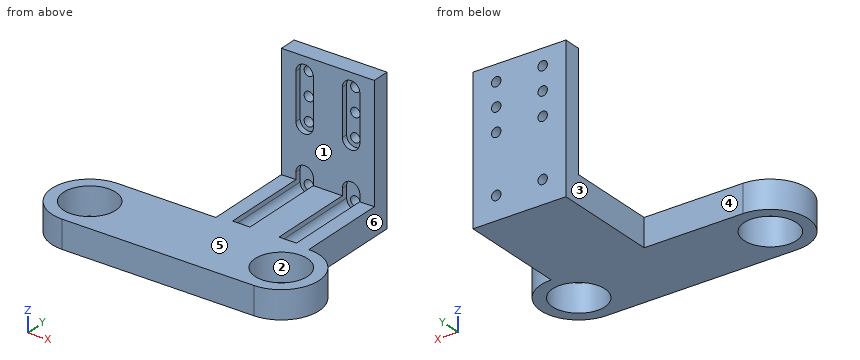
Autodesk Inventor part; units mm, degrees
ref_plane "Work Plane1" through (1.5875, 73.0746, 0) normal (0, 1, 0) x (1, 0, 0)
ref_plane "YZ Plane" through (0, 0, 0) normal (1, 0, 0) x (0, 1, 0)
ref_plane "XZ Plane" through (0, 0, 0) normal (0, 1, 0) x (-1, 0, 0)
sketch "Sketch1" plane through (0, 0, 0) normal (0, 0, 1) x (1, 0, 0)
  line L0 (-52.3875, 0) -> (52.3875, 0) construction
  line L1 (-52.3875, -20.6502) -> (52.3875, -20.6502)
  line L2 (52.3875, 20.6502) -> (-52.3875, 20.6502)
  arc A0 (-52.3875, 20.6502) -> (-52.3875, -20.6502) centre (-52.3875, 0) ccw
  arc A1 (52.3875, -20.6502) -> (52.3875, 20.6502) centre (52.3875, 0) ccw
  point P0 (0, 0)
  dimension "d0" = 104.775
  dimension "d1" = 20.6502
extrude "Extrusion1" add sketch "Sketch1" along normal blind 15.24
sketch "Sketch2" plane through (0, 0, 15.24) normal (0, 0, 1) x (1, 0, 0)
  arc A0 (-52.3875, 20.6502) -> (-52.3875, -20.6502) centre (-52.3875, 0) ccw
  circle A1 centre (-52.3875, 0) radius 14.3002
  arc A2 (52.3875, -20.6502) -> (52.3875, 20.6502) centre (52.3875, 0) ccw
  circle A3 centre (52.3875, 0) radius 14.3002
  point P0 (0, 0)
  dimension "d4" = 28.6004
extrude "Extrusion2" cut sketch "Sketch2" against normal through all
sketch "Sketch3" plane through (0, 0, 15.24) normal (0, 0, 1) x (1, 0, 0)
  line L0 (1.5875, 79.4246) -> (52.3875, 79.4246)
  line L1 (52.3875, 79.4246) -> (52.3875, 20.6502)
  line L2 (52.3875, 20.6502) -> (1.5875, 20.6502)
  line L3 (1.5875, 20.6502) -> (1.5875, 79.4246)
  line L4 (52.3875, 20.6502) -> (-52.3875, 20.6502)
  circle A0 centre (26.9875, 101.6496) radius 7.0281
  circle A1 centre (52.3875, 0) radius 14.3002
  point P0 (0, 0)
  point P1 (26.9875, 20.6502)
  point P2 (26.9875, 79.4246)
  dimension "d7" = 50.8
  dimension "d8" = 22.225
  dimension "d9" = 104.775
  dimension "d10" = 79.4246
extrude "Extrusion3" add sketch "Sketch3" against normal up to surface (15.24 mm away) contours L0 L1 L2 L3
sketch "Sketch4" plane through (0, 0, 15.24) normal (0, 0, 1) x (1, 0, 0)
  line L0 (1.5875, 79.4246) -> (1.5875, 20.6502)
  line L1 (1.5875, 79.4246) -> (52.3875, 79.4246)
  line L2 (52.3875, 79.4246) -> (52.3875, 69.8996)
  line L3 (52.3875, 69.8996) -> (1.5875, 69.8996)
  line L4 (1.5875, 69.8996) -> (1.5875, 79.4246)
  line L5 (52.3875, 20.6502) -> (52.3875, 79.4246)
  point P0 (0, 0)
  point P1 (25.4, 20.6502)
  dimension "d13" = 9.525
extrude "Extrusion4" add sketch "Sketch4" along normal blind 63.5
sketch "Sketch5" plane through (1.5875, 79.4246, 0) normal (0, 1, 0) x (1, 0, 0)
  circle A0 centre (38.1, -12.7) radius 2.5797
  line L0 (0, 0) -> (50.8, 0)
  line L1 (50.8, 0) -> (50.8, -78.74)
  circle A1 centre (12.7, -12.7) radius 2.5797
  circle A2 centre (38.1, -44.45) radius 2.5797
  circle A3 centre (12.7, -44.45) radius 2.5797
  circle A4 centre (38.1, -57.15) radius 2.5797
  circle A5 centre (12.7, -57.15) radius 2.5797
  circle A6 centre (38.1, -69.85) radius 2.5797
  circle A7 centre (12.7, -69.85) radius 2.5797
  line L2 (25.4, 0) -> (25.4, -6.0461)
  dimension "d17" = 5.1594
  dimension "d18" = 12.7
  dimension "d21" = 25.4
  dimension "d24" = 31.75
  dimension "d29" = 12.7
  dimension "d51" = 12.7
extrude "Extrusion5" cut sketch "Sketch5" against normal blind 50.8
ref_plane "Work Plane1" through (1.5875, 73.0746, 0) normal (0, 1, 0) x (1, 0, 0)
sketch "Sketch6" plane through (1.5875, 73.0746, 0) normal (0, 1, 0) x (1, 0, 0)
  line L0 (-53.975, 0) -> (50.8, 0)
  line L1 (50.8, -15.24) -> (50.8, -78.74)
  line L2 (38.1, -12.7) -> (38.1, -19.05) construction
  line L3 (33.3375, -12.7) -> (33.3375, -19.05)
  line L4 (42.8625, -19.05) -> (42.8625, -12.7)
  arc A0 (42.8625, -12.7) -> (33.3375, -12.7) centre (38.1, -12.7) ccw
  arc A1 (33.3375, -19.05) -> (42.8625, -19.05) centre (38.1, -19.05) ccw
  line L5 (12.7, -12.7) -> (12.7, -19.05) construction
  line L6 (7.9375, -12.7) -> (7.9375, -19.05)
  line L7 (17.4625, -19.05) -> (17.4625, -12.7)
  arc A2 (17.4625, -12.7) -> (7.9375, -12.7) centre (12.7, -12.7) ccw
  arc A3 (7.9375, -19.05) -> (17.4625, -19.05) centre (12.7, -19.05) ccw
  circle A4 centre (38.1, -44.45) radius 2.5797 construction
  circle A5 centre (38.1, -69.85) radius 2.5797 construction
  line L8 (38.1, -44.45) -> (38.1, -69.85) construction
  line L9 (33.3375, -44.45) -> (33.3375, -69.85)
  line L10 (42.8625, -69.85) -> (42.8625, -44.45)
  arc A6 (42.8625, -44.45) -> (33.3375, -44.45) centre (38.1, -44.45) ccw
  arc A7 (33.3375, -69.85) -> (42.8625, -69.85) centre (38.1, -69.85) ccw
  circle A8 centre (12.7, -44.45) radius 2.5797 construction
  circle A9 centre (12.7, -69.85) radius 2.5797 construction
  line L11 (12.7, -44.45) -> (12.7, -69.85) construction
  line L12 (7.9375, -44.45) -> (7.9375, -69.85)
  line L13 (17.4625, -69.85) -> (17.4625, -44.45)
  arc A10 (17.4625, -44.45) -> (7.9375, -44.45) centre (12.7, -44.45) ccw
  arc A11 (7.9375, -69.85) -> (17.4625, -69.85) centre (12.7, -69.85) ccw
  circle A12 centre (38.1, -12.7) radius 2.5797 construction
  circle A13 centre (12.7, -12.7) radius 2.5797 construction
  point P0 (-1.5875, 0)
  point P1 (38.1, -15.875)
  point P2 (12.7, -15.875)
  point P3 (38.1, -57.15)
  point P4 (12.7, -57.15)
  dimension "d47" = 6.35
  dimension "d48" = 4.7625
extrude "Extrusion6" cut sketch "Sketch6" against normal blind 50.8
properties part number "IntakeChainLinkVP"
Read the model definition and answer for the solid it produces. Units are mm, in the model's axes. Face numbers are marked on the shaded views. A direction names the side the tool comes from. Coordinates: 2 decimals unless noted, no trailing zeros. Write each loop counter-clockwise with the first axis right and the second up, starting at its lowest first coordinate (ties: lowest second). Pieces come first, ordered by that corner, then holes. Notation, with made-up numbers: (65.25, 55.25) - (78.25, 55.25) arc R19 ccw to (78.25, 92.25) - close; hole circle Ø7 at (-33, 6.25). An arc over 180 degrees is marked (long way). Answer as a JSON object with one key per item and string values. Group by question number.
1. A cutting plane is placed at A-A (y = 0). Determine the outline of the cut face in (x, z), plus the area to 3 significant figures.
2. Consider L1, parallel to X at y = 78, z = 44; L2, parallel to X at y = 76.25, z = 69.85; L3, parallel to Y at x = 18.5, z = 39. Determine where each line is inside the solid, lowest interval first. Write a range as [from, to].
3. Each of these flat-tipped pins is pushed along its axis until it touches: P1, Ø6.5, axis at x = 39.69, z = 69.85, coming from the -Y side; P2, Ø3, axis at y = 31.5, z = 13.5, coming from the -X side; P3, Ø1, axis at x = 32.5, z = 60.5, coming from the -Y side; P4, Ø3, axis at x = 13.5, z = 56.5, coming from the -Y side. Where does it stop, or does it pass through?
4. A cutting plane is placed at D-D (x = -15.5). Determine the outline of the cut face in (y, z), plus the area to 3 significant figures.
5. The mould has two halves that part along X. Classify the marked faces 1, 2 and 3: +X half, -X half, draft (parallel to the pull), parting line (faces both ways), or undercut.
6. A cutting plane is placed at B-B (z = 57.15). Give the number of separate pieces and of enclosed holes in the cut face, plus the area to 3 significant figures.
7. Which of the six approach directions +Z, -Z, +X, -X, +Y, -Y give full straight-line access (tool end or side, diameter ignored) to the marked faces 4, 5 and 6?
Worked out:
{
 "1": {"outline": "(-73.04, 0) - (-66.69, 0) - (-66.69, 15.24) - (-73.04, 15.24) - close; (-38.09, 0) - (38.09, 0) - (38.09, 15.24) - (-38.09, 15.24) - close; (66.69, 0) - (73.04, 0) - (73.04, 15.24) - (66.69, 15.24) - close", "area": "1,350 mm²"},
 "2": {"L1": "x = [1.59, 11.75], [16.83, 37.15], [42.23, 52.39]", "L2": "x = [1.59, 11.71], [16.87, 37.11], [42.27, 52.39]", "L3": "y = [69.9, 79.42]"},
 "3": {"P1": "stops at y = 73.07", "P2": "stops at x = 1.59", "P3": "stops at y = 69.9", "P4": "passes through"},
 "4": {"outline": "(-20.65, 0) - (20.65, 0) - (20.65, 15.24) - (-20.65, 15.24) - close", "area": "629 mm²"},
 "5": {"face 1": "draft", "face 2": "undercut", "face 3": "-X half"},
 "6": {"separate pieces": "3", "enclosed holes": "0", "area": "358 mm²"},
 "7": {"face 4": "+Z, -Z, -X, +Y", "face 5": "+Z, +X, -X, -Y", "face 6": "+Z, -Z, +X, +Y"}
}
